```python
from build123d import *

# Parameters (mm, degrees)
F1_R     = 12.7
F5_R     = 6.35
F6_DEPTH = 32.810532029


with BuildPart() as f2:
    # F2: sweep along a path in F0
    with BuildLine(Plane.XY) as f2_path:
        Line((0, 0), (76.2, 0))
        ThreePointArc((76.2, 0), (112.1210244843, 14.8789755157), (127, 50.8))
        Line((127, 50.8), (127, 127))
    # F1 (on Right) → F2 (sweep)
    with BuildSketch(Plane.YZ):
        Circle(F1_R)
    sweep(path=f2_path.line)

    # F5 (on plane+point) → F6 (join, through all)
    with BuildSketch(Plane.XZ.offset(19.5012806053)):
        with Locations((121.1012806053, 0)):
            Circle(F5_R)
    extrude(amount=-F6_DEPTH)


solid = f2.part
```
The listing builds one solid part. Answer for the finished solid, in the listing's coordinates (mm). A direction names the side the tool comes from. Coordinates: 2 decimals unless noted, no trailing zeros. Order: outer loops, then holes, each group sorted by start corner. A loop starts at its lowest first (then second) coordinate and runs counter-clockwise, first axis right, second up. Notation, with made-up numbers: M 29,-23 L 79,-23 A17 ccw 79,-6 Z; hole C -7,29.5 d7. An arc over 180 degrees is marked long. Answer as a JSON object with one key per item and string values. Group by question number.
1. Section C-C on x = 65 is taken. Write down the section's boundary in (y, z).
2. A tool of negligible diameter and unlimited length cuts with its end or side. For faces 4 (the flat face through (127, 127, 0)), 5 (the cylindrical face through (139.688, 89.433, 0.558)), from which of +Z, -Z, +X, -X, +Y, -Y can it reach the whole face along a straight path? Write none if from no direction.
3. Section A-A on z = 0 is taken. Write down the section's boundary in (x, y), then the cut area to 3 significant figures.
4. Section D-D on z = 11 is taken. Write down the section's boundary in (x, y), then the cut area to 3 significant figures.
5. Straight lines are drawn through the part: line 1 (X direction, y = -3, z = 4.25); line 2 (X direction, y = -6.5, z = -5); line 3 (Z direction, x = 59, y = -1). For each, find the intervals that lie inside material, in ascending order.
6. Section B-B on y = 114.5 is taken. Write down the section's boundary in (x, z), then the cut area to 3 significant figures.
7. Determine the mould class of faces 1 (the flat face through (0, 0, 0)), 2 (the cylindrical face through (38.63, -2.75, -12.4)), 3 (the cylindrical face through (127.158, -6.971, 1.907)) for opening direction X: released by +X, released by -X, zero draft, split by the parting line, or undercut.
8. Flat-ended cylindrical pins translate along their axes: P1, Ø1, axis at y = 109, z = -7.5, coming from the -X side; P2, Ø1.5, axis at y = -4.5, z = -4, coming from the +X side; P3, Ø1, axis at x = 19, z = -3, coming from the -Y side; P4, Ø8, axis at y = 108, z = -4, coming from the +X side. Find the tip coordinate at first contact, or state that the pin passes through.
Values follow:
{
 "1": {"outline": "C 0,0 d25.4"},
 "2": {"face 4": "+Z, -Z, +X, -X, +Y", "face 5": "+Y"},
 "3": {"outline": "M 0,-12.7 L 76.2,-12.7 A63.5 ccw 114.75,0.34 L 114.75,-19.5 L 127.45,-19.5 L 127.45,13.31 A63.5 ccw 139.7,50.8 L 139.7,127 L 114.3,127 L 114.3,50.8 A38.1 cw 76.2,12.7 L 0,12.7 Z", "area": "6,220 mm2"},
 "4": {"outline": "M 0,-6.35 L 76.2,-6.35 A57.15 ccw 133.35,50.8 L 133.35,127 L 120.65,127 L 120.65,50.8 A44.45 cw 76.2,6.35 L 0,6.35 Z", "area": "2,950 mm2"},
 "5": {"line 1": "0 to 108.53, 116.38 to 125.82", "line 2": "0 to 101.09, 117.19 to 125.02", "line 3": "-12.66 to 12.66"},
 "6": {"outline": "C 127,0 d25.4", "area": "507 mm2"},
 "7": {"face 1": "released by -X", "face 2": "zero draft", "face 3": "undercut"},
 "8": {"P1": "x = 116.4", "P2": "x = 126.56", "P3": "y = -12.45", "P4": "x = 139.7"}
}
